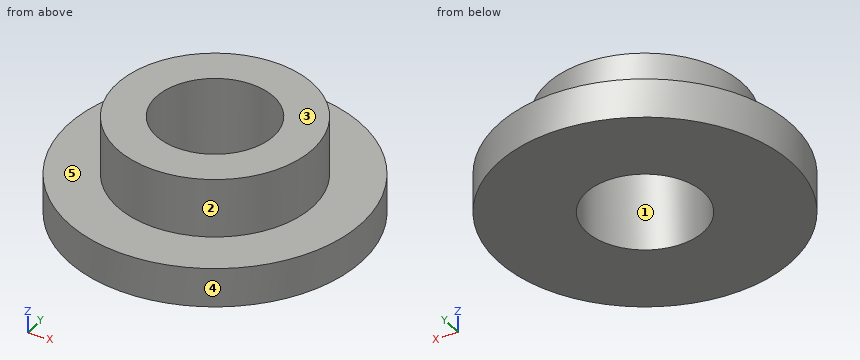
Autodesk Inventor part; units mm, degrees
ref_plane "YZ Plane" through (0, 0, 0) normal (1, 0, 0) x (0, 1, 0)
ref_plane "XZ Plane" through (0, 0, 0) normal (0, 1, 0) x (-1, 0, 0)
ref_plane "XY Plane" through (0, 0, 0) normal (0, 0, 1) x (1, 0, 0)
sketch "スケッチ1" plane through (0, 0, 0) normal (0, 0, 1) x (1, 0, 0)
  circle A0 centre (0, 0) radius 5
  circle A1 centre (0, 0) radius 7.5
  dimension "d0" = 10
  dimension "d1" = 15
extrude "押し出し1" add sketch "スケッチ1" along normal blind 8 contours A0 | A1
sketch "スケッチ2" plane through (0, 0, 8) normal (0, 0, 1) x (1, 0, 0)
  circle A0 centre (0, 0) radius 5
  circle A1 centre (0, 0) radius 3
  circle A2 centre (0, 0) radius 10
  dimension "d4" = 10
  dimension "d5" = 6
  dimension "d8" = 20
extrude "押し出し2" cut sketch "スケッチ2" against normal blind 6
sketch "スケッチ4" plane through (0, 0, 2) normal (0, 0, 1) x (1, 0, 0)
  circle A0 centre (0, 0) radius 3
extrude "押し出し4" cut sketch "スケッチ4" against normal blind 5
sketch "スケッチ5" plane through (0, 0, 8) normal (0, 0, 1) x (1, 0, 0)
  circle A0 centre (0, 0) radius 10.699
extrude "押し出し5" cut sketch "スケッチ5" against normal blind 3
properties part number "10mm_bearing"
Source: CAD feature listing. Evaluate the final solid. Frame: model axes, mm. Face numbers are marked on the shaded views. A direction names the side the tool comes from. Coordinates: 2 decimals unless noted, no trailing zeros. Loops run counter-clockwise (first coordinate to the right, second up) from the corner with the lowest first, then second, coordinate; pieces in that order, holes last. Notation, with made-up numbers: M -31,-32 L -12,-32 A26 ccw -12,-11 Z; hole C 35,-19.75 d7. An arc over 180 degrees is marked long. Put each result on its own line as item: value. Start each with the question number.
1) Cut plane A-A on y = 0. Return the cut outline in (x, z).
2) Ray query, L1, parallel to Y at x = 0, z = 3.9; L2, parallel to Z at x = -4.5, y = 5.5; L3, parallel to X at y = 2.5, z = 3.6. Return the intervals inside material, ascending. Write a range as from..to.
3) Cut plane C-C on z = 1.4. Return the cut outline in (x, y), then the cut area to 3 significant figures.
4) Cut plane D-D on x = -3.5. Return the cut outline in (y, z), then the cut area to 3 significant figures.
5) Reachability of the marked faces 4 and 5 from +Z, -Z, +X, -X, +Y, -Y: full face, straight path, thin tool, end or side. Return the list, or none.
6) Pull-direction query (Y, two-part tool) for the marked faces 1, 2 and 3; classes: pulls with the +Y half, pulls with the -Y half, needs draft (parallel to the pull), parting line crosses it, or undercut.
7) Contact query for flat-ended pins moving along their axis: pin 1 Ø1.5 at (x, z) = (-5.5, 2) entering from +Y; pin 2 Ø1 at (x, y) = (-4, -4.5) entering from +Z; pin 3 Ø1.5 at (x, z) = (-1.5, 0.5) entering from +Y. Output: stop coordinate, or through.
The answers:
1. outline: M -7.5,0 L -3,0 L -3,5 L -5,5 L -5,2 L -7.5,2 Z; M 3,0 L 7.5,0 L 7.5,2 L 5,2 L 5,5 L 3,5 Z
2. L1: y = -5..-3, 3..5
2. L2: z = 0..2
2. L3: x = -4.33..-1.66, 1.66..4.33
3. outline: C 0,0 d15; hole C 0,0 d6
3. area: 148 mm²
4. outline: M -6.63,0 L 6.63,0 L 6.63,2 L 3.57,2 L 3.57,5 L -3.57,5 L -3.57,2 L -6.63,2 Z
4. area: 48.0 mm²
5. face 4: +Z, -Z
5. face 5: +Z
6. face 1: undercut
6. face 2: parting line crosses it
6. face 3: needs draft
7. pin 1: stops at y = 5.8
7. pin 2: stops at z = 2
7. pin 3: stops at y = 7.46
